Input: part model. Units: mm. Frame: model coordinates. A direction names the side the tool comes from. Round coordinates to 2 decimals unless told otherwise and drop trailing zeros. Order: outer loops, then holes, each group sorted by start corner. A loop starts at its lowest first (then second) coordinate and runs counter-clockwise, first axis right, second up. Notation, with made-up numbers: (-9.75, 44.25) -> (39.25, 44.25) arc R19 ccw to (39.25, 78.25) -> close; hole circle Ø5 at (75, 25.5). An arc over 180 degrees is marked (long way). Answer as CSV lines item,"result". Start each with the question number.
1) Access query for faces 4 (the face through (6.77, -15.7, 71.84)), 5 (the face through (70, 39.5, 15)), 6 (the face through (-1, 112.5, 12)), 7 (the face through (66, 63.5, 52)), 8 (the face through (80, -52.5, 30)). Directions: +Z, -Z, +X, -X, +Y, -Y. A direction counts if a zero-diameter tool reaches every point of the face in a straight line with its end or side. Return the directions, or none.
2) Section query A-A, the plane y = -82.5. Output: boundary loops of the cut face in (x, z).
3) Line query: L1, parallel to Y at x = 75, z = 6.25; L2, parallel to X at y = -82, z = 27; L3, parallel to Z at x = -77, y = -85. Output: solid intervals per line, ascending.
4) Section query D-D, the plane y = 56. Output: boundary loops of the cut face in (x, z).
5) First-contact query: P1, Ø4, axis at x = -69.5, y = -78, coming from the +Z side; P2, Ø22, axis at x = 67, z = 13, coming from the -Y side; P3, Ø4, axis at x = -73, y = -5.5, coming from the +Z side. Flat tips, straight axial feed; report the tip coordinate or a pass-through.
6) Section query B-B, the plane x = 75. Output: boundary loops of the cut face in (y, z), and give its area (3 significant figures).
7) Mould query, pull axis X, two halves, no side actions, for faces 1 (the face through (102.15, -109.49, 17.74)), 2 (the face through (71.748, -97.143, 30.07)), 3 (the face through (-71, -72, 54)). Classes: +X half, -X half, draft (parallel to the pull), parting line (faces both ways), or undercut.
8) Section query C-C, the plane z = 11. Output: boundary loops of the cut face in (x, y).
```python
from build123d import *

# Parameters (mm, degrees)
F0_W            = 210
F0_H            = 225
F1_DEPTH        = 25
F3_DEPTH        = 95
F4_R            = 37.5
F5_DEPTH        = 10
F5_DEPTH_BACK   = 127.1
F6_R            = 40
F7_DEPTH        = 10
F7_DEPTH_BACK   = 127.1
F8_W            = 60
F8_H            = 60
F9_DEPTH        = 10
F10_R           = 10
F12_DEPTH       = 20
F14_D           = 15
F14_CBORE_D     = 30
F14_CBORE_DEPTH = 10
F15_R           = 10
F16_R           = 19.5
F17_DEPTH       = 235.001
F18_R           = 19.5
F19_DEPTH       = 220.001
F20_SIZE        = 2
F21_R           = 10


with BuildPart() as f1:
    # F0 (on Top) → F1 (new body)
    with BuildSketch(Plane.XY):
        Rectangle(F0_W, F0_H)
    extrude(amount=F1_DEPTH)

    # F2 (on face) → F3 (join)
    with BuildSketch(Plane.XY.offset(25)):
        with BuildLine():
            Line((-71, -32.5), (-71, -112.5))
            Line((-71, -112.5), (-56, -112.5))
            Line((-56, -112.5), (-56, -46.481817))
            ThreePointArc((-56, -46.481817), (7.488853, -14.988853), (38.981817, 48.5))
            Line((38.981817, 48.5), (105, 48.5))
            Line((105, 48.5), (105, 63.5))
            Line((105, 63.5), (25, 63.5))
            ThreePointArc((25, 63.5), (-3.117749, -4.382251), (-71, -32.5))
        make_face()
    extrude(amount=F3_DEPTH)

    # F4 (on face) → F5 (join, two sides)
    with BuildSketch(Plane.XZ.offset(112.5)) as f5_sk:
        with Locations((-63.5, 120)):
            Circle(F4_R)
    extrude(amount=F5_DEPTH)
    extrude(f5_sk.sketch, amount=-F5_DEPTH_BACK)

    # F6 (on face) → F7 (join, two sides)
    with BuildSketch(Plane.YZ.offset(105)) as f7_sk:
        with Locations((56, 120)):
            Circle(F6_R)
    extrude(amount=F7_DEPTH)
    extrude(f7_sk.sketch, amount=-F7_DEPTH_BACK)

    # F8 (on face) → F9 (join)
    with BuildSketch(Plane.XY.offset(25)):
        with Locations((75, -82.5)):
            Rectangle(F8_W, F8_H)
    extrude(amount=F9_DEPTH)

    # F10
    f10_edges = [f1.edges().sort_by_distance(p)[0] for p in [
        (45, -52.5, 30),
    ]]
    fillet(f10_edges, radius=F10_R)

    # F11 (on face) → F12 (cut)
    with BuildSketch(Plane.XY.offset(25)):
        with BuildLine():
            ThreePointArc((46.575508, 39.5), (13.852814, -21.352814), (-47, -54.075508))
            Line((-47, -54.075508), (-47, -103.5))
            Line((-47, -103.5), (36, -103.5))
            Line((36, -103.5), (36, -62.5))
            ThreePointArc((36, -62.5), (41.564971, -49.064971), (55, -43.5))
            Line((55, -43.5), (96, -43.5))
            Line((96, -43.5), (96, 39.5))
            Line((96, 39.5), (46.575508, 39.5))
        make_face()
    extrude(amount=-F12_DEPTH, mode=Mode.SUBTRACT)

    # F14 (through all)
    with Locations(Plane.XY.offset(35)):
        with Locations((75, -82.5)):
            CounterBoreHole(F14_D / 2, F14_CBORE_D / 2, F14_CBORE_DEPTH)

    # F15
    f15_edges = [f1.edges().sort_by_distance(p)[0] for p in [
        (-47, -54.075508, 15),
        (46.575508, 39.5, 15),
        (-47, -103.5, 15),
        (36, -103.5, 15),
        (96, -43.5, 15),
        (96, 39.5, 15),
    ]]
    fillet(f15_edges, radius=F15_R)

    # F16 (on face) → F17 (cut, through all)
    with BuildSketch(Plane.XZ.offset(122.5)):
        with Locations((-63.5, 120)):
            Circle(F16_R)
    extrude(amount=-F17_DEPTH, mode=Mode.SUBTRACT)

    # F18 (on face) → F19 (cut, through all)
    with BuildSketch(Plane.YZ.offset(115)):
        with Locations((56, 120)):
            Circle(F18_R)
    extrude(amount=-F19_DEPTH, mode=Mode.SUBTRACT)

    # F20
    f20_edges = [f1.edges().sort_by_distance(p)[0] for p in [
        (115, 36.5, 120),
        (-83, -122.5, 120),
        (-83, 14.6, 120),
        (-22.1, 36.5, 120),
    ]]
    chamfer(f20_edges, length=F20_SIZE)

    # F21
    f21_edges = [f1.edges().sort_by_distance(p)[0] for p in [
        (-105, 112.5, 12.5),
        (105, 112.5, 12.5),
        (105, -112.5, 17.5),
        (-105, -112.5, 12.5),
    ]]
    fillet(f21_edges, radius=F21_R)


solid = f1.part
```
Findings:
1,face 4,"+X, -Y"
1,face 5,"none"
1,face 6,"+Z, -Z, +X, -X, +Y"
1,face 7,"+X, -X, +Y"
1,face 8,"+Z, +X"
2,outline,"(-105, 0) -> (67.5, 0) -> (67.5, 25) -> (60, 25) -> (60, 35) -> (45, 35) -> (45, 25) -> (36, 25) -> (36, 5) -> (-47, 5) -> (-47, 25) -> (-56, 25) -> (-56, 83.26) arc R37.5 ccw (long way) to (-71, 83.26) -> (-71, 25) -> (-105, 25) -> close; (82.5, 0) -> (105, 0) -> (105, 35) -> (90, 35) -> (90, 25) -> (82.5, 25) -> close; hole circle Ø39 at (-63.5, 120)"
3,L1,"y = -112.5 to -90, -75 to -43.5, 39.5 to 112.5"
3,L2,"x = -71 to -56, 45 to 60.01, 89.99 to 105"
3,L3,"z = 0 to 25, 85.01 to 105.93, 134.07 to 154.99"
4,outline,"(-105, 0) -> (105, 0) -> (105, 80) -> (115, 80) -> (115, 98.5) -> (113, 100.5) -> (-20.1, 100.5) -> (-22.1, 98.5) -> (-22.1, 80) -> (24.71, 80) -> (24.71, 25) -> (-105, 25) -> close; (-22.1, 141.5) -> (-20.1, 139.5) -> (113, 139.5) -> (115, 141.5) -> (115, 160) -> (-22.1, 160) -> close"
5,P1,"stops at z = 157.29"
5,P2,"stops at y = -112.5"
5,P3,"stops at z = 156.74"
6,outline,"(-112.5, 0) -> (-90, 0) -> (-90, 25) -> (-97.5, 25) -> (-97.5, 35) -> (-112.5, 35) -> close; (-75, 0) -> (112.5, 0) -> (112.5, 25) -> (63.5, 25) -> (63.5, 80.71) arc R40 ccw (long way) to (48.5, 80.71) -> (48.5, 25) -> (39.5, 25) -> (39.5, 5) -> (-43.5, 5) -> (-43.5, 25) -> (-52.5, 25) -> (-52.5, 35) -> (-67.5, 35) -> (-67.5, 25) -> (-75, 25) -> close; hole circle Ø39 at (56, 120)"
6,area,"8,550 mm^2"
7,face 1,"+X half"
7,face 2,"undercut"
7,face 3,"-X half"
8,outline,"(-105, -102.5) arc R10 ccw to (-95, -112.5) -> (95, -112.5) arc R10 ccw to (105, -102.5) -> (105, 102.5) arc R10 ccw to (95, 112.5) -> (-95, 112.5) arc R10 ccw to (-105, 102.5) -> close; hole (-47, -93.5) arc R10 ccw to (-37, -103.5) -> (26, -103.5) arc R10 ccw to (36, -93.5) -> (36, -62.5) arc R19 cw to (55, -43.5) -> (86, -43.5) arc R10 ccw to (96, -33.5) -> (96, 29.5) arc R10 ccw to (86, 39.5) -> (54.48, 39.5) arc R10 ccw to (44.82, 32.12) arc R120 cw to (-39.62, -52.32) arc R10 ccw to (-47, -61.98) -> close; hole circle Ø15 at (75, -82.5)"
